CAD build for the part. Positions are in the model's coordinates, mm. Face numbers are marked on the shaded views. A direction names the side the tool comes from. Give positions to 0.01 mm unless a question says otherwise; leave off trailing zeros. Loops run counter-clockwise (first coordinate to the right, second up) from the corner with the lowest first, then second, coordinate; pieces in that order, holes last.
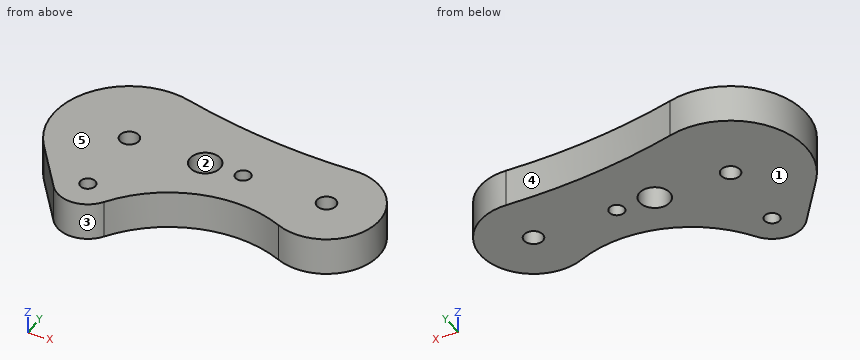
```python
from build123d import *

# Parameters (mm, degrees)
SKETCH1_R           = 1.25
SKETCH1_R_2         = 2
SKETCH1_R_3         = 1
BOSS_EXTRUDE1_DEPTH = 5


with BuildPart() as part:
    # Sketch1 → Boss-Extrude1 (new body)
    with BuildSketch(Plane.XY):
        with BuildLine():
            Line((-8, -6), (-3.2, -12.4))
            ThreePointArc((-3.2, -12.4), (0.118790152, -13.998235723), (3.336840869, -12.205786258))
            ThreePointArc((3.336840869, -12.205786258), (12.188123784, -5.673630591), (23.164757844, -6.400109524))
            ThreePointArc((23.164757844, -6.400109524), (32.870759027, -1.338906415), (25.775337581, 6.996393842))
            ThreePointArc((25.775337581, 6.996393842), (14.14827012, 7.469801361), (2.712885779, 9.624980559))
            ThreePointArc((2.712885779, 9.624980559), (-8.247629875, 5.654785711), (-8, -6))
        make_face()
        Circle(SKETCH1_R, mode=Mode.SUBTRACT)
        with Locations((26, 0)):
            Circle(SKETCH1_R, mode=Mode.SUBTRACT)
        with Locations((10, 0)):
            Circle(SKETCH1_R_2, mode=Mode.SUBTRACT)
        with Locations((15, 0)):
            Circle(SKETCH1_R_3, mode=Mode.SUBTRACT)
        with Locations((0, -10)):
            Circle(SKETCH1_R_3, mode=Mode.SUBTRACT)
    extrude(amount=BOSS_EXTRUDE1_DEPTH)


solid = part.part
```
1. Probe line 1 along Y through (x, z) = (0, 2.85); line 2 along X through (y, z) = (-0.5, 3.2); line 3 along Y through (x, z) = (15, 3.55). List the from-to ranges inside material, lowest first.
Responses:
line 1: y = -14 to -11, -9 to -1.25, 1.25 to 10
line 2: x = -9.99 to -1.15, 1.15 to 8.06, 11.94 to 14.13, 15.87 to 24.85, 27.15 to 32.98
line 3: y = -5.12 to -1, 1 to 7.38
2. Pull direction Y, two halves, no side cores. Call the marked faces 1, 2 and 3: released by +Y, released by -Y, zero draft, split by the parting line, or undercut.
Responses:
face 1: zero draft
face 2: undercut
face 3: released by -Y
3. Saw through at C-C, the plane x = 9.5. List the corners of the cut face in (y, z).
Responses:
outline: (-6.73, 0) - (-1.94, 0) - (-1.94, 5) - (-6.73, 5) - close; (1.94, 0) - (8.14, 0) - (8.14, 5) - (1.94, 5) - close
4. Drop a flat-ended pin along its axis: pin 1 (1 mm diameter, centred on x = -5.5, z = 2, fed in from -Y). Give the stop position or say it passes through.
Responses:
pin 1: stops at y = -10
5. Saw through at B-B, the plane x = 0. List the corners of the cut face in (y, z), and give its area (3 significant figures).
Responses:
outline: (-14, 0) - (-11, 0) - (-11, 5) - (-14, 5) - close; (-9, 0) - (-1.25, 0) - (-1.25, 5) - (-9, 5) - close; (1.25, 0) - (10, 0) - (10, 5) - (1.25, 5) - close
area: 97.5 mm2
6. Saw through at D-D, the plane y = -10. List the corners of the cut face in (x, z), and give its area (3 significant figures).
Responses:
outline: (-5, 0) - (-1, 0) - (-1, 5) - (-5, 5) - close; (1, 0) - (5.09, 0) - (5.09, 5) - (1, 5) - close
area: 40.5 mm2
7. Saw through at A-A, the plane y = 0. List the corners of the cut face in (x, z).
Responses:
outline: (-10, 0) - (-1.25, 0) - (-1.25, 5) - (-10, 5) - close; (1.25, 0) - (8, 0) - (8, 5) - (1.25, 5) - close; (12, 0) - (14, 0) - (14, 5) - (12, 5) - close; (16, 0) - (24.75, 0) - (24.75, 5) - (16, 5) - close; (27.25, 0) - (33, 0) - (33, 5) - (27.25, 5) - close
8. Tool access for the marked faces 4 and 5: list every direction of +Z, -Z, +X, -X, +Y, -Y with a clear straight run to the whole face (end or side of a thin tool).
Responses:
face 4: +Z, -Z, +Y
face 5: +Z, +X, -X, +Y, -Y
